```python
from build123d import *

# Parameters (mm, degrees)
F1_DEPTH = 25.4
F2_DEPTH = 7.9375
F0_W     = 31.585604
F0_H     = 28.575
F4_DEPTH = 63.5


with BuildPart() as f1:
    # F0 (on Front) → F1 (new body, symmetric)
    with BuildSketch(Plane.XZ):
        Polygon((60.325, 66.675), (60.325, 61.9252), (60.325, 42.8752), (60.325, 38.1), (79.539396, 38.1), (79.539396, 66.675), align=None)
        with BuildLine():
            Line((22.225, 9.525), (41.275, 9.525))
            Line((41.275, 9.525), (41.275, 27.0002))
            ThreePointArc((41.275, 27.0002), (45.92468, 38.22552), (57.15, 42.8752))
            Line((57.15, 42.8752), (60.325, 42.8752))
            Line((60.325, 42.8752), (60.325, 61.9252))
            Line((60.325, 61.9252), (57.15, 61.9252))
            add(Edge.make_bspline(
                [(53.857929, 61.769697), (54.939593, 61.830793), (56.036819, 61.882698), (57.15, 61.9252)],
                knots=[109.332626, 109.332626, 109.332626, 109.332626, 111.504536, 111.504536, 111.504536, 111.504536], degree=3))
            ThreePointArc((53.857929, 61.769697), (31.31658, 50.503179), (22.225, 27.0002))
            Line((22.225, 27.0002), (22.225, 9.525))
        make_face()
    extrude(amount=F1_DEPTH, both=True)

    # F0 (on Front) → F2 (join, symmetric)
    with BuildSketch(Plane.XZ):
        with BuildLine():
            add(Edge.make_bspline(
                [(-41.275, 9.525), (-15.607869, 32.326474), (-0.592367, 58.694147), (53.857929, 61.769697)],
                knots=[0, 0, 0, 0, 109.332626, 109.332626, 109.332626, 109.332626], degree=3))
            Line((-41.275, 9.525), (22.225, 9.525))
            Line((22.225, 9.525), (22.225, 27.0002))
            ThreePointArc((22.225, 27.0002), (31.31658, 50.503179), (53.857929, 61.769697))
        make_face()
    extrude(amount=F2_DEPTH, both=True)

    # F0 (on Front) → F3 (revolve)
    with BuildSketch(Plane.XZ):
        with Locations((95.332198, 52.3875)):
            Rectangle(F0_W, F0_H)
    revolve(axis=Axis((79.539396, 0, 52.3875), (0, 0, 1)))

    # F0 (on Front) → F4 (join, symmetric)
    with BuildSketch(Plane.XZ):
        Polygon((-41.275, 9.525), (-41.275, -9.525), (41.275, -9.525), (41.275, 9.525), (22.225, 9.525), align=None)
    extrude(amount=F4_DEPTH, both=True)


solid = f1.part
```
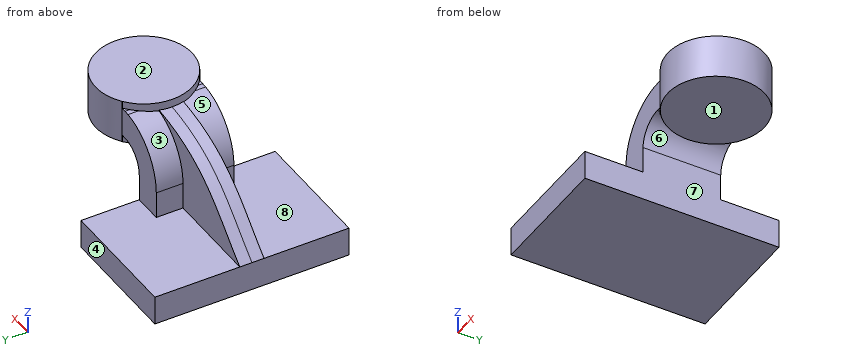
Geometry: final body of the model. Coordinates: model frame, mm. Face numbers are marked on the shaded views. A direction names the side the tool comes from. Round coordinates to 2 decimals unless told otherwise and drop trailing zeros. Order: outer loops, then holes, each group sorted by start corner. A loop starts at its lowest first (then second) coordinate and runs counter-clockwise, first axis right, second up. Notation, with made-up numbers: (89, 68) - (94, 68) arc R13 cw to (94, 85) - close; hole circle Ø2 at (-38.75, -20). An arc over 180 degrees is marked (long way). Use CSV: the item, a comma, the result in double quotes. Start each with the question number.
Q1. First-contact query: pin 1 (14 mm diameter, centred on y = 17, z = 18.5, fed in from -X) (3 decimals); pin 2 (11.5 mm diameter, centred on x = 36, z = 28, fed in from +Y); pin 3 (8 mm diameter, centred on x = 24, z = 34, fed in from -Y); pin 4 (8 mm diameter, centred on y = 32, z = 23, fed in from +X). Flat tips, straight axial feed; report the tip coordinate or a pass-through.
Q2. Access query for the marked faces 1, 2, 3, 4 and 5. Directions: +Z, -Z, +X, -X, +Y, -Y. A direction counts if a zero-diameter tool reaches every point of the face in a straight line with its end or side. Return the directions, or none.
Q3. Section query B-B (z = -0.5). Return loops of the section in (x, y) (3 decimals).
Q4. Section query A-A (y = 46.5). Return loops of the section in (x, z) (3 decimals).
Q5. Mould query, pull axis X, two halves, no side actions, for the marked faces 6, 7 and 8. Classes: +X half, -X half, draft (parallel to the pull), parting line (faces both ways), or undercut.
Q6. Material intervals for line 1 along Z through (x, y) = (101.5, -2) (3 decimals); line 2 along X through (y, z) = (7, 38.5); line 3 along Z through (x, y) = (13, -10) (3 decimals), sorted ascending. Write a range as from..to.
Result set:
1,pin 1,"stops at x = 22.225"
1,pin 2,"stops at y = 25.4"
1,pin 3,"stops at y = -25.4"
1,pin 4,"passes through"
2,face 1,"-Z, +X, +Y, -Y"
2,face 2,"+Z, +X, -X, +Y, -Y"
2,face 3,"+Z, -X, +Y"
2,face 4,"+Z, -Z, +X, -X, +Y"
2,face 5,"+Z, -X, -Y"
3,outline,"(-41.275, -63.5) - (41.275, -63.5) - (41.275, 63.5) - (-41.275, 63.5) - close"
4,outline,"(-41.275, -9.525) - (41.275, -9.525) - (41.275, 9.525) - (-41.275, 9.525) - close"
5,face 6,"undercut"
5,face 7,"+X half"
5,face 8,"draft"
6,line 1,"z = 38.1..66.675"
6,line 2,"x = -10.44..46.21, 48.74..110.34"
6,line 3,"z = -9.525..9.525"
